```python
from build123d import *

# Parameters (mm, degrees)
BOSS_EXTRUDE1_DEPTH = 18
CUT_EXTRUDE1_DEPTH  = 4


with BuildPart() as part:
    # Sketch1 → Boss-Extrude1 (new body)
    with BuildSketch(Plane(origin=(0, 0, 0), x_dir=(1, 0, 0), z_dir=(0, 1, 0))):
        with BuildLine():
            Line((47.5, 30), (57.5, 30))
            Line((57.5, 30), (57.5, 70))
            Line((57.5, 70), (42.5, 70))
            Line((42.5, 70), (42.5, 35))
            Line((42.5, 35), (37.5, 35))
            ThreePointArc((37.5, 35), (-16.783008589, 13.550775542), (-40, -40))
            Line((-40, -40), (-35, -40))
            ThreePointArc((-35, -40), (-13.247474683, 10.015241636), (37.5, 30))
            Line((37.5, 30), (47.5, 30))
        make_face()
    extrude(amount=BOSS_EXTRUDE1_DEPTH)

    # Sketch4 → Cut-Extrude1 (cut)
    with BuildSketch(Plane(origin=(0, 0, 0), x_dir=(-1, 0, 0), z_dir=(0, -1, 0))):
        Polygon((-50, 70), (-45, 70), (-45, 40), (-55, 40), (-55, 70), align=None)
    extrude(amount=-CUT_EXTRUDE1_DEPTH, mode=Mode.SUBTRACT)


solid = part.part
```
Work out the finished part from the listing and answer in its coordinate system (mm). A direction names the side the tool comes from. Coordinates: 2 decimals unless noted, no trailing zeros. Loops run counter-clockwise (first coordinate to the right, second up) from the corner with the lowest first, then second, coordinate; pieces in that order, holes last. Notation, with made-up numbers: (52, 34.25) - (76, 34.25) arc R26 ccw to (76, 64.25) - close; hole circle Ø11 at (-1, 58.5). An arc over 180 degrees is marked (long way). Use a Markdown table: item, result.
Item 1: Find section A-A, the plane z = -59. Determine the outline of the cut face in (x, y).
Evaluation:
| item | result |
|---|---|
| outline | (42.5, 0) - (45, 0) - (45, 4) - (55, 4) - (55, 0) - (57.5, 0) - (57.5, 18) - (42.5, 18) - close |
Item 2: Given pin 1 Ø8 at (y, z) = (9, 26) entering from -X; pin 2 Ø4.5 at (x, y) = (49, 2) entering from -Z; pin 3 Ø3 at (x, z) = (51.5, -51) entering from -Y; pin 4 Ø1.5 at (x, y) = (41, 9) entering from -Z, each flat-ended and moving along its own axis, determine where each tip first touches the part or whether it passes through.
Evaluation:
| item | result |
|---|---|
| pin 1 | stops at x = -39.18 |
| pin 2 | stops at z = -70 |
| pin 3 | stops at y = 4 |
| pin 4 | stops at z = -35 |
Item 3: Consider probe 1 along X at (y, z) = (6, -58.5); probe 2 along Z at (x, y) = (46, 10.25); probe 3 along Y at (x, z) = (46, -53). Determine where each line is inside the solid, lowest interval first. Write a range as from..to.
Evaluation:
| item | result |
|---|---|
| probe 1 | x = 42.5..57.5 |
| probe 2 | z = -70..-30 |
| probe 3 | y = 4..18 |
Item 4: Find section D-D, the plane z = 6. Determine the outline of the cut face in (x, y).
Evaluation:
| item | result |
|---|---|
| outline | (-31.37, 0) - (-25.68, 0) - (-25.68, 18) - (-31.37, 18) - close |
Item 5: Find section C-C, the plane x = 39. Determine the outline of the cut face in (y, z).
Evaluation:
| item | result |
|---|---|
| outline | (0, -35) - (18, -35) - (18, -30) - (0, -30) - close |
Item 6: The mould has two halves that part along X. Classify faces 1 (the flat face through (42.5, 9, -53)), 2 (the flat face through (57.5, 9, -50)), 3 (the flat face through (50, 4, -55)), 4 (the flat face through (-38, 9, 40)): +X half, -X half, draft (parallel to the pull), parting line (faces both ways), or undercut.
Evaluation:
| item | result |
|---|---|
| face 1 | -X half |
| face 2 | +X half |
| face 3 | undercut |
| face 4 | draft |
Item 7: For faces 5 (the flat face through (47, 9, -30)), 6 (the flat face through (40, 9, -35)), 7 (the flat face through (55, 2, -55)), determine the directions among +Z, -Z, +X, -X, +Y, -Y from which every point of the face is accessible in a straight line to the end or side of a thin tool.
Evaluation:
| item | result |
|---|---|
| face 5 | +Z, +X, +Y, -Y |
| face 6 | -Z, -X, +Y, -Y |
| face 7 | -Z, -Y |
Item 8: Find section B-B, the plane y = 13. Determine the outline of the cut face in (x, z).
Evaluation:
| item | result |
|---|---|
| outline | (-40, 40) arc R76.26 ccw to (37.5, -35) - (42.5, -35) - (42.5, -70) - (57.5, -70) - (57.5, -30) - (37.5, -30) arc R71.26 cw to (-35, 40) - close |
